Autodesk Inventor part; units mm, degrees
ref_plane "Work Plane1" through (-16.5, 0, 0) normal (1, 0, 0) x (0, 0, -1)
ref_plane "YZ Plane" through (0, 0, 0) normal (1, 0, 0) x (0, 1, 0)
ref_plane "XZ Plane" through (0, 0, 0) normal (0, 1, 0) x (-1, 0, 0)
sketch "Sketch1" plane through (0, 0, 0) normal (0, 1, 0) x (-1, 0, 0)
  line L0 (0, 0) -> (33, 0)
  line L1 (33, 0) -> (33, -10)
  line L2 (33, -10) -> (0, -10)
  line L3 (0, -10) -> (0, 0)
  dimension "d0" = 33
  dimension "d1" = 10
extrude "Extrusion1" add sketch "Sketch1" along normal blind 4
sketch "Sketch2" plane through (0, 4, 0) normal (0, 1, 0) x (1, 0, 0)
  circle A0 centre (-5.343, 5) radius 1.8
  point P0 (0, 0)
  dimension "d9" = 3.6
extrude "Extrusion2" cut sketch "Sketch2" against normal blind 4
ref_plane "Work Plane1" through (-16.5, 0, 0) normal (1, 0, 0) x (0, 0, -1)
mirror "Mirror1" about plane through (-16.5, 0, 0) normal (1, 0, 0) of "Extrusion2"
fillet "Fillet1" radius 3 4 edges at (-33, 2, 0) (-33, 2, -10) (0, 2, 0) (0, 2, -10)
sketch "Sketch3" plane through (0, 4, 0) normal (0, 1, 0) x (1, 0, 0)
  line L0 (-30, 0) -> (-3, 0)
  line L1 (-30, 10) -> (-3, 10)
  line L2 (-20, 0) -> (-13, 0)
  line L3 (-13, 0) -> (-13, 10)
  line L4 (-13, 10) -> (-20, 10)
  line L5 (-20, 10) -> (-20, 0)
  point P0 (0, 0)
  dimension "d10" = 7
  dimension "d11" = 10
extrude "Extrusion3" add sketch "Sketch3" along normal blind 0.3
sketch "Sketch4" plane through (0, 4, 0) normal (0, 1, 0) x (1, 0, 0)
  line L0 (-3, 0) -> (-8, 0)
  line L1 (-8, 0) -> (-8, 10)
  line L2 (-8, 10) -> (-3, 10)
  line L3 (0, 7) -> (0, 3)
  arc A0 (-3, 0) -> (0, 3) centre (-3, 3) ccw
  arc A1 (0, 7) -> (-3, 10) centre (-3, 7) ccw
  circle A2 centre (-5.343, 5) radius 1.8
  circle A3 centre (-5.343, 5) radius 1.8
  point P0 (0, 0)
  point P1 (0, 10)
  dimension "d14" = 8
  dimension "d15" = 10
  dimension "d16" = 3
extrude "Extrusion4" add sketch "Sketch4" along normal blind 0.3
mirror "Mirror2" about plane through (-16.5, 0, 0) normal (1, 0, 0) of "Extrusion4"
sketch "Sketch6" plane through (0, 4.3, 0) normal (0, 1, 0) x (1, 0, 0)
  line L0 (-20, 0) -> (-13, 0)
  line L1 (-20, 0) -> (-18.2027, 0)
  line L2 (-18.2027, 0) -> (-18.2027, -0.8691)
  line L3 (-18.2027, -0.8691) -> (-20, -0.8691)
  line L4 (-20, -0.8691) -> (-20, 0)
  point P0 (0, 0)
extrude "Extrusion6" add sketch "Sketch6" against normal up to surface (4.3 mm away)
sketch "Sketch7" plane through (0, 4.3, 0) normal (0, 1, 0) x (1, 0, 0)
  line L0 (-13, 0) -> (-13, 10)
  line L1 (-13, 0) -> (-14.8092, 0)
  line L2 (-14.8092, 0) -> (-14.8092, -0.8691)
  line L3 (-14.8092, -0.8691) -> (-13, -0.8691)
  line L4 (-13, -0.8691) -> (-13, 0)
  point P0 (0, 0)
extrude "Extrusion7" add sketch "Sketch7" against normal up to surface (4.3 mm away)
properties part number "8 peristaltic pump clamp 0.3mm"
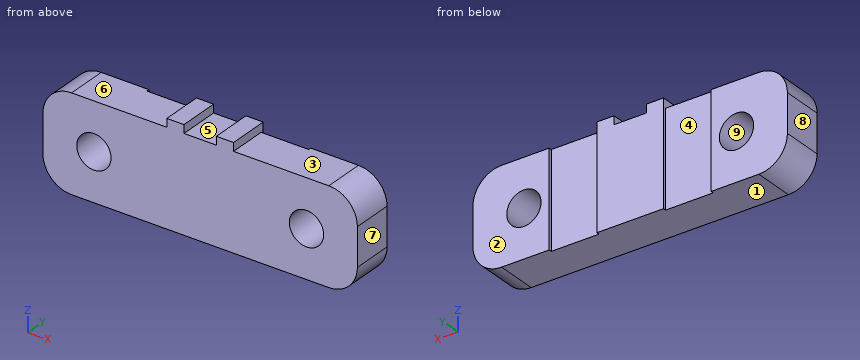
Input: part model. Units: mm. Frame: model coordinates. Face numbers are marked on the shaded views. A direction names the side the tool comes from. Round coordinates to 2 decimals unless told otherwise and drop trailing zeros. Loops run counter-clockwise (first coordinate to the right, second up) from the corner with the lowest first, then second, coordinate; pieces in that order, holes last. Notation, with made-up numbers: (52, -11) -> (102, -11) arc R28 ccw to (102, 21) -> close; hole circle Ø4 at (30, 49). An arc over 180 degrees is marked (long way). One line per item, written item: value.
(1) Material intervals for line 1 (X direction, y = 2.85, z = -5); line 2 (Z direction, x = -27.5, y = 2.4); line 3 (Y direction, x = -21, z = -2.25), sorted ascending. Write a range as [from, to].
Geometry check:
line 1: [-33, -29.46], [-25.86, -7.14], [-3.54, 0]
line 2: [-10, -6.79], [-3.21, 0]
line 3: [0, 4]
(2) Section D-D (x = -28.5). Return the cut outline in (y, z).
Geometry check:
outline: (0, -10) -> (4.3, -10) -> (4.3, -6.59) -> (0, -6.59) -> close; (0, -3.41) -> (4.3, -3.41) -> (4.3, 0) -> (0, 0) -> close
(3) Set-up query: the marked faces 1, 2, 3, 4 and 5. Return all of +Z, -Z, +X, -X, +Y, -Y with unobstructed straight access to the full face (end or side cutting, diameter ignored); none if empty.
Geometry check:
face 1: -Z, +X, -X, +Y, -Y
face 2: +Z, -Z, +X, -X, +Y
face 3: +Z, +X, +Y, -Y
face 4: +Z, -Z, +Y
face 5: +Z, +Y, -Y
(4) Section B-B (x = -6). Return the cut outline in (y, z).
Geometry check:
outline: (0, -10) -> (4.3, -10) -> (4.3, -6.68) -> (0, -6.68) -> close; (0, -3.32) -> (4.3, -3.32) -> (4.3, 0) -> (0, 0) -> close
(5) Mould query, pull axis X, two halves, no side actions, for the marked faces 6, 7, 8 and 9. Classes: pulls with the +X half, pulls with the -X half, needs draft (parallel to the pull), parting line crosses it, or undercut.
Geometry check:
face 6: needs draft
face 7: pulls with the +X half
face 8: pulls with the -X half
face 9: undercut
(6) Section A-A (z = -5). Return the cut outline in (x, y).
Geometry check:
outline: (-33, 0) -> (-29.46, 0) -> (-29.46, 4.3) -> (-33, 4.3) -> close; (-25.86, 0) -> (-7.14, 0) -> (-7.14, 4.3) -> (-8, 4.3) -> (-8, 4) -> (-13, 4) -> (-13, 4.3) -> (-20, 4.3) -> (-20, 4) -> (-25, 4) -> (-25, 4.3) -> (-25.86, 4.3) -> close; (-3.54, 0) -> (0, 0) -> (0, 4.3) -> (-3.54, 4.3) -> close
(7) Section C-C (y = 2.3). Return the cut outline in (x, z).
Geometry check:
outline: (-33, -7) arc R3 ccw to (-30, -10) -> (-3, -10) arc R3 ccw to (0, -7) -> (0, -3) arc R3 ccw to (-3, 0) -> (-13, 0) -> (-13, 0.87) -> (-14.81, 0.87) -> (-14.81, 0) -> (-18.2, 0) -> (-18.2, 0.87) -> (-20, 0.87) -> (-20, 0) -> (-30, 0) arc R3 ccw to (-33, -3) -> close; hole circle Ø3.6 at (-27.66, -5); hole circle Ø3.6 at (-5.34, -5)
(8) Pin query (flat end, axial travel): pin 1 (2.5 mm diameter, centred on x = -23.5, z = -4.5, fed in from +Y); pin 2 (3 mm diameter, centred on x = -5.343, z = -5, fed in from +Y); pin 3 (1.3 mm diameter, centred on x = -8.5, y = 1.5, fed in from +Z). Return the tip coordinate at first contact, or that it passes through.
Geometry check:
pin 1: y = 4
pin 2: through
pin 3: z = 0
